Verification items for the finished model (mm, model axes). A direction names the side the tool comes from. Give positions to 0.01 mm unless a question says otherwise; leave off trailing zeros. Write each loop counter-clockwise with the first axis right and the second up, starting at its lowest first coordinate (ties: lowest second). Pieces come first, ordered by that corner, then holes. Notation, with made-up numbers: (4, 36.5) -> (38, 36.5) arc R23 ccw to (38, 64.5) -> close; hole circle Ø5 at (13, 1.5). An arc over 180 degrees is marked (long way). Use one line per item in the form item = value. Start each with the question number.
(1) Section check B-B, the plane z = 2. Record the cut outline in (x, y), plus the area to 3 significant figures.
(2) Depth check by flat-ended pin: pin 1 Ø11 at (x, y) = (34.5, 23.5) entering from +Z; pin 2 Ø0.8 at (x, y) = (21.5, 28.5) entering from +Z; pin 3 Ø3 at (x, z) = (26.5, 36.5) entering from -Y. Enter the tip coordinate at first touch or a pass-through.
(3) Section check A-A, the plane y = 3.5. Record the cut outline in (x, z).
(4) Section check D-D, the plane z = 22. Record the cut outline in (x, y).
(5) Set-up check for faces 4 (the face through (35, 15, 5)), 5 (the face through (35, 20, 10)), 6 (the face through (20, 29, 21)), 7 (the face through (11, 32, 40)), 8 (the face through (35, 35, 20)): record each of +Z, -Z, +X, -X, +Y, -Y from which the full face is reachable in a straight line by a thin tool's end or side.
(6) Release check for a two-part mould opening along Y. For faces 1 (the face through (20, 20, 0)), 2 (the face through (21, 30, 21)), 3 (the face through (27, 30, 37)) record: pulls with the +Y half, pulls with the -Y half, needs draft (parallel to the pull), parting line crosses it, or undercut.
(7) Section check C-C, the plane x = 31. Record the cut outline in (y, z), plus the area to 4 significant figures.
(8) Scan lines: L1, parallel to Z at x = 37, y = 18.5; L2, parallel to Z at x = 7, y = 5.5. Record each from-to range of solid material in increasing order.
from build123d import *

# Parameters (mm, degrees)
SKETCH1_W            = 40
SKETCH1_H            = 40
BOSS_EXTRUDE1_DEPTH  = 20
CUT_EXTRUDE1_DEPTH   = 20
BOSS_EXTRUDE2_DEPTH  = 10
BOSS_EXTRUDE3_DEPTH  = 10
SKETCH5_W            = 10
SKETCH5_H            = 12.477634561
BOSS_EXTRUDE4_DEPTH  = 20
BOSS_EXTRUDE5_DEPTH  = 10
SKETCH7_W            = 30
SKETCH7_H            = 10
BOSS_EXTRUDE6_DEPTH  = 20
BOSS_EXTRUDE7_DEPTH  = 10
BOSS_EXTRUDE8_DEPTH  = 20
SKETCH13_W           = 10
SKETCH13_H           = 10
BOSS_EXTRUDE10_DEPTH = 10
BOSS_EXTRUDE13_DEPTH = 10
SKETCH15_W           = 20
SKETCH15_H           = 30.380258446
BOSS_EXTRUDE15_DEPTH = 30
CUT_EXTRUDE2_DEPTH   = 30
CUT_EXTRUDE3_DEPTH   = 30
CUT_EXTRUDE4_DEPTH   = 30
CUT_EXTRUDE5_DEPTH   = 30
BOSS_EXTRUDE16_DEPTH = 10
CUT_EXTRUDE6_DEPTH   = 10
SKETCH25_W           = 10
SKETCH25_H           = 10
CUT_EXTRUDE7_DEPTH   = 10


with BuildPart() as part:
    # Sketch1 → Boss-Extrude1 (new body)
    with BuildSketch(Plane.XY):
        with Locations((20, 20)):
            Rectangle(SKETCH1_W, SKETCH1_H)
    extrude(amount=BOSS_EXTRUDE1_DEPTH)

    # Sketch2 → Cut-Extrude1 (cut)
    with BuildSketch(Plane.XY.offset(20)):
        Polygon((20, 10), (20, 0), (40, 0), (40, 30), align=None)
    extrude(amount=-CUT_EXTRUDE1_DEPTH, mode=Mode.SUBTRACT)

    # Sketch3 → Boss-Extrude2 (add)
    with BuildSketch(Plane.XZ):
        Polygon((20, 20), (0, 20), (0, 30), (10, 30), align=None)
    extrude(amount=-BOSS_EXTRUDE2_DEPTH)

    # Sketch4 → Boss-Extrude3 (add)
    with BuildSketch(Plane(origin=(20, 0, 0), x_dir=(0, 0, -1), z_dir=(1, 0, 0))):
        Polygon((0, 0), (-20, 10), (0, 10), align=None)
    extrude(amount=BOSS_EXTRUDE3_DEPTH)

    # Sketch5 → Boss-Extrude4 (add)
    with BuildSketch(Plane.XY.offset(20)):
        with Locations((25, 16.238817281)):
            Rectangle(SKETCH5_W, SKETCH5_H)
    extrude(amount=-BOSS_EXTRUDE4_DEPTH)

    # Sketch6 → Boss-Extrude5 (add)
    with BuildSketch(Plane(origin=(0, 0, 0), x_dir=(-1, 0, 0), z_dir=(0, 0, -1))):
        Polygon((-30, 10), (-40, 20), (-40, 30), (-30, 20), align=None)
    extrude(amount=-BOSS_EXTRUDE5_DEPTH)

    # Sketch7 → Boss-Extrude6 (add)
    with BuildSketch(Plane.XY.offset(20)):
        with Locations((15, 35)):
            Rectangle(SKETCH7_W, SKETCH7_H)
    extrude(amount=BOSS_EXTRUDE6_DEPTH)

    # Sketch8 → Boss-Extrude7 (add)
    with BuildSketch(Plane.ZY):
        Polygon((40, 30), (40, 20), (30, 10), (20, 10), (20, 30), align=None)
    extrude(amount=-BOSS_EXTRUDE7_DEPTH)

    # Sketch9 → Boss-Extrude8 (add)
    with BuildSketch(Plane.XY.offset(40)):
        Polygon((10, 20), (20, 30), (10, 30), align=None)
    extrude(amount=-BOSS_EXTRUDE8_DEPTH)

    # Sketch13 → Boss-Extrude10 (add)
    with BuildSketch(Plane(origin=(0, 40, 0), x_dir=(1, 0, 0), z_dir=(0, 1, 0))):
        with Locations((35, -25)):
            Rectangle(SKETCH13_W, SKETCH13_H)
    extrude(amount=-BOSS_EXTRUDE10_DEPTH)

    # Sketch12 → Boss-Extrude13 (add)
    with BuildSketch(Plane(origin=(10, -10, 10), x_dir=(-0.816496581, -0.40824829, 0.40824829), z_dir=(-0.577350269, 0.577350269, -0.577350269))):
        Polygon((-12.247448714, 21.213203436), (0, 42.426406871), (-12.247448714, 49.497474683), (-24.494897428, 28.284271247), align=None)
    extrude(amount=BOSS_EXTRUDE13_DEPTH)

    # Sketch15 → Boss-Extrude15 (add)
    with BuildSketch(Plane(origin=(0, 40, 0), x_dir=(1, 0, 0), z_dir=(0, 1, 0))):
        with Locations((10, -24.809870777)):
            Rectangle(SKETCH15_W, SKETCH15_H)
    extrude(amount=-BOSS_EXTRUDE15_DEPTH)

    # Sketch17 → Cut-Extrude2 (cut)
    with BuildSketch(Plane(origin=(10, -10, 10), x_dir=(-0.816496581, -0.40824829, 0.40824829), z_dir=(-0.577350269, 0.577350269, -0.577350269))):
        Polygon((-12.247448714, 49.497474683), (0, 42.426406871), (-12.247448714, 21.213203436), align=None)
    extrude(amount=-CUT_EXTRUDE2_DEPTH, mode=Mode.SUBTRACT)

    # Sketch18 → Cut-Extrude3 (cut)
    with BuildSketch(Plane(origin=(10, -10, 10), x_dir=(-0.816496581, -0.40824829, 0.40824829), z_dir=(-0.577350269, 0.577350269, -0.577350269))):
        Polygon((0, 42.426406871), (0, 28.284271247), (-12.247448714, 21.213203436), align=None)
    extrude(amount=-CUT_EXTRUDE3_DEPTH, mode=Mode.SUBTRACT)

    # Sketch20 → Cut-Extrude4 (cut)
    with BuildSketch(Plane(origin=(0, 0, 0), x_dir=(-0.365148372, -0.182574186, -0.912870929), z_dir=(0.816496581, 0.40824829, -0.40824829))):
        Polygon((-32.86335345, 4.472135955), (-43.8178046, 2.236067977), (-43.8178046, 13.416407865), align=None)
    extrude(amount=-CUT_EXTRUDE4_DEPTH, mode=Mode.SUBTRACT)

    # Sketch21 → Cut-Extrude5 (cut)
    with BuildSketch(Plane.ZY):
        Polygon((30, 10), (40, 20), (40, 10), align=None)
    extrude(amount=-CUT_EXTRUDE5_DEPTH, mode=Mode.SUBTRACT)

    # Sketch23 → Boss-Extrude16 (add)
    with BuildSketch(Plane(origin=(10, -10, 10), x_dir=(-0.816496581, -0.40824829, 0.40824829), z_dir=(-0.577350269, 0.577350269, -0.577350269))):
        Polygon((-12.247448714, 49.497474683), (-24.494897428, 28.284271247), (-36.742346142, 35.355339059), align=None)
    extrude(amount=BOSS_EXTRUDE16_DEPTH)

    # Sketch24 → Cut-Extrude6 (cut)
    with BuildSketch(Plane(origin=(0, 40, 0), x_dir=(1, 0, 0), z_dir=(0, 1, 0))):
        Polygon((30, -30), (40, -20), (40, -30), align=None)
    extrude(amount=-CUT_EXTRUDE6_DEPTH, mode=Mode.SUBTRACT)

    # Sketch25 → Cut-Extrude7 (cut)
    with BuildSketch(Plane(origin=(0, 40, 0), x_dir=(1, 0, 0), z_dir=(0, 1, 0))):
        with Locations((35, -25)):
            Rectangle(SKETCH25_W, SKETCH25_H)
    extrude(amount=-CUT_EXTRUDE7_DEPTH, mode=Mode.SUBTRACT)


solid = part.part
Completed:
q1.outline = (0, 0) -> (20, 0) -> (20, 1) -> (30, 1) -> (30, 10) -> (40, 20) -> (40, 40) -> (0, 40) -> close
q1.area = 1,440 mm²
q2.pin_1 = 26.78
q2.pin_2 = 37.57
q2.pin_3 = 30
q3.outline = (0, 0) -> (30, 0) -> (30, 7) -> (20, 7) -> (20, 20) -> (10, 30) -> (0, 30) -> close
q4.outline = (0, 0) -> (18, 0) -> (18, 10) -> (38, 30) -> (30, 30) -> (30, 40) -> (0, 40) -> close; hole (20, 29.32) -> (20.68, 30) -> (20, 30) -> close
q5.face_4 = +Z, -Z, +X, -Y
q5.face_5 = +Z, +X, -Y
q5.face_6 = none
q5.face_7 = +Z, +X, -X, +Y, -Y
q5.face_8 = +Z, +X, +Y
q6.face_1 = needs draft
q6.face_2 = undercut
q6.face_3 = pulls with the -Y half
q7.outline = (11, 0) -> (40, 0) -> (40, 20) -> (30, 20) -> (30, 29) -> (21, 20) -> (21, 10) -> (11, 10) -> close
q7.area = 520.5 mm²
q8.L1 = 0 to 10
q8.L2 = 0 to 30
